Check sheet for the modelled part. Datum: model origin and axes. Units: mm. Give positions to 0.01 mm unless a question says otherwise; leave off trailing zeros. Write each loop counter-clockwise with the first axis right and the second up, starting at its lowest first coordinate (ties: lowest second). Pieces come first, ordered by that corner, then holes. Notation, with made-up numbers: (-27, -12) -> (-11, -12) arc R10 ccw to (-11, -1) -> close; hole circle Ø4 at (64.5, 5). An arc over 180 degrees is marked (long way). Use a Markdown table: item, result. Add a question column.
1. Scan lines: probe 1 along X at (y, z) = (46.25, 0); probe 2 along Y at (x, z) = (143, 1); probe 3 along Y at (x, z) = (185, -18.5). Record each from-to range of solid material in increasing order. Write a range as [from, to].
2. Release check for a two-part mould opening along Z. For faces 1 (the cylindrical face through (148, 45, 0)), 2 (the flat face through (0, 45.1, -2.3)), 3 (the cylindrical face through (147.9, 46.997, -0.517)) record: released by +Z, released by -Z, zero draft, split by the parting line, or undercut.
3. Gauge pin test, flat ends, axial feed: P1, Ø2, axis at x = 32, z = 0, coming from the +Y side; P2, Ø2, axis at x = 233.5, y = 39.5, coming from the +Z side; P3, Ø1, axis at x = 144, y = 33.5, coming from the +Z side; P4, Ø4, axis at x = 217, y = 45, coming from the -Z side. Record the tip position at first contact, or that the pin passes through.
4. Cross-section at A-A (x = 111.5). Enter the section's corners in (y, z).
5. Cross-section at B-B (z = -15). Enter the section's corners in (x, y).
from build123d import *

# Parameters (mm, degrees)
BOSS_EXTRUDE1_DEPTH = 300
SKETCH3_R           = 1.75
CUT_EXTRUDE1_DEPTH  = 306.897117362


with BuildPart() as part:
    # Sketch1 → Boss-Extrude1 (new body)
    with BuildSketch(Plane(origin=(0, 0, 0), x_dir=(0, 0, -1), z_dir=(1, 0, 0))):
        with BuildLine():
            Line((31.819805153, 31.819805153), (33.234018716, 33.234018716))
            ThreePointArc((33.234018716, 33.234018716), (0, 47), (-33.234018716, 33.234018716))
            Line((-33.234018716, 33.234018716), (-31.819805153, 31.819805153))
            ThreePointArc((-31.819805153, 31.819805153), (0, 45), (31.819805153, 31.819805153))
        make_face()
    extrude(amount=BOSS_EXTRUDE1_DEPTH)

    # Sketch3 → Cut-Extrude1 (cut, through all)
    with BuildSketch(Plane(origin=(0, 0, -3.698980221), x_dir=(1, 0, 0), z_dir=(0, 1, 0))):
        with Locations(Location((7, -3.698980221, 0), (0, 0, 90))):
            Circle(SKETCH3_R)
        with Locations(Location((32, -3.698980221, 0), (0, 0, 90))):
            Circle(SKETCH3_R)
    extrude(amount=CUT_EXTRUDE1_DEPTH, mode=Mode.SUBTRACT)


solid = part.part
Worked answers:
| question | item | result |
|---|---|---|
| 1 | probe 1 | x = [0, 5.25], [8.75, 30.25], [33.75, 300] |
| 1 | probe 2 | y = [44.99, 46.99] |
| 1 | probe 3 | y = [41.02, 43.21] |
| 2 | face 1 | undercut |
| 2 | face 2 | zero draft |
| 2 | face 3 | split by the parting line |
| 3 | P1 | passes through |
| 3 | P2 | stops at z = 26.96 |
| 3 | P3 | stops at z = 33.23 |
| 3 | P4 | stops at z = -18.97 |
| 4 | outline | (31.82, -31.82) -> (33.23, -33.23) arc R47 ccw to (33.23, 33.23) -> (31.82, 31.82) arc R45 cw to start |
| 5 | outline | (0, 42.43) -> (300, 42.43) -> (300, 44.54) -> (0, 44.54) -> close |
